Work out the finished part from the listing and answer in its coordinate system (mm). Face numbers are marked on the shaded views. A direction names the side the tool comes from. Give positions to 0.01 mm unless a question says otherwise; leave off trailing zeros. Order: outer loops, then holes, each group sorted by start corner. A loop starts at its lowest first (then second) coordinate and runs counter-clockwise, first axis right, second up. Notation, with made-up numbers: (-27, 5) - (-9, 5) arc R19 cw to (-9, 12) - close; hole circle Ø1 at (17.5, 63). An arc over 180 degrees is marked (long way). Put each result on its own line as item: value.
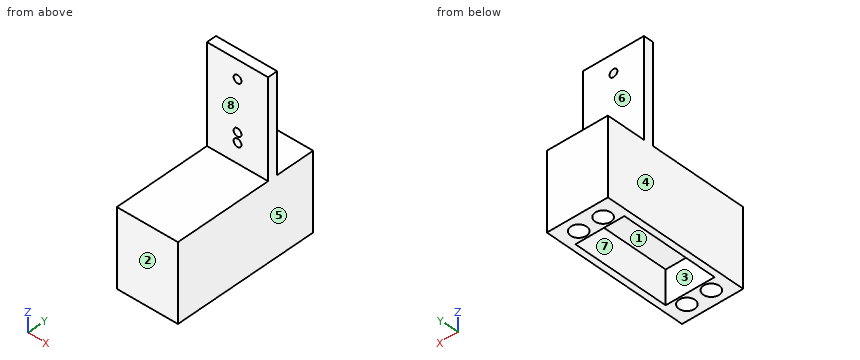
```python
from build123d import *

# Parameters (mm, degrees)
SKETCH1_W           = 27.5
SKETCH1_H           = 40
BOSS_EXTRUDE1_DEPTH = 12.5
SKETCH2_W           = 5.015
SKETCH2_H           = 40.03
SKETCH2_W_2         = 10
CUT_EXTRUDE1_DEPTH  = 13.765
SKETCH6_R           = 3.25
CUT_EXTRUDE2_DEPTH  = 12
SKETCH7_R           = 1.6
CUT_EXTRUDE3_DEPTH  = 61.763887302


with BuildPart() as part:
    # Sketch1 → Boss-Extrude1 (new, symmetric)
    with BuildSketch(Plane(origin=(0, 0, 0), x_dir=(0, 0, -1), z_dir=(1, 0, 0))):
        with Locations((17.75, 20)):
            Rectangle(SKETCH1_W, SKETCH1_H)
        Polygon((0, -10), (0, 30), (-40, 30), (-40, 34), (0, 34), (0, 50), (31.5, 50), (31.5, 40), (4, 40), (4, 0), (31.5, 0), (31.5, -10), align=None)
    extrude(amount=BOSS_EXTRUDE1_DEPTH, both=True)

    # Sketch2 → Cut-Extrude1 (cut, symmetric)
    with BuildSketch(Plane(origin=(0, 0, -31.5), x_dir=(-1, 0, 0), z_dir=(0, 0, -1))):
        with Locations((7.5075, 20)):
            Rectangle(SKETCH2_W, SKETCH2_H)
        with Locations((0, 20)):
            Rectangle(SKETCH2_W_2, SKETCH2_H)
        with Locations((-7.5075, 20)):
            Rectangle(SKETCH2_W, SKETCH2_H)
    extrude(amount=CUT_EXTRUDE1_DEPTH, both=True, mode=Mode.SUBTRACT)

    # Sketch6 → Cut-Extrude2 (cut)
    with BuildSketch(Plane(origin=(0, 0, -31.5), x_dir=(-1, 0, 0), z_dir=(0, 0, -1))):
        with Locations(Location((-5, 44, 0), (0, 0, 90))):
            Circle(SKETCH6_R)
        with Locations(Location((5, 44, 0), (0, 0, 90))):
            Circle(SKETCH6_R)
        with Locations(Location((5, -4, 0), (0, 0, 90))):
            Circle(SKETCH6_R)
        with Locations(Location((-5, -4, 0), (0, 0, 90))):
            Circle(SKETCH6_R)
    extrude(amount=-CUT_EXTRUDE2_DEPTH, mode=Mode.SUBTRACT)

    # Sketch7 → Cut-Extrude3 (cut, through all)
    with BuildSketch(Plane(origin=(0, 34, 0), x_dir=(1, 0, 0), z_dir=(0, 1, 0))):
        with Locations(Location((0, -32.5, 0), (0, 0, 270))):
            Circle(SKETCH7_R)
        with Locations(Location((0, -12, 0), (0, 0, 270))):
            Circle(SKETCH7_R)
        with Locations(Location((0, -8, 0), (0, 0, 270))):
            Circle(SKETCH7_R)
    extrude(amount=-CUT_EXTRUDE3_DEPTH, mode=Mode.SUBTRACT)


solid = part.part
```
(1) A tool of negligible diameter and unlimited length cuts with its end or side. For the marked faces 5, 6, 7 and 8, from which of +Z, -Z, +X, -X, +Y, -Y can it reach the whole face along a straight path? Write none if from no direction.
Geometry check:
face 5: +Z, -Z, +X, +Y, -Y
face 6: +Z, +X, -X, +Y
face 7: -Z
face 8: +Z, +X, -X, -Y
(2) Section D-D, the plane x = -5 is taken. Write down the section's boundary in (y, z) (3 decimals).
Geometry check:
outline: (-10, -31.5) - (-7.25, -31.5) - (-7.25, -19.5) - (-0.75, -19.5) - (-0.75, -31.5) - (-0.015, -31.5) - (-0.015, -17.735) - (40.015, -17.735) - (40.015, -31.5) - (40.75, -31.5) - (40.75, -19.5) - (47.25, -19.5) - (47.25, -31.5) - (50, -31.5) - (50, 0) - (34, 0) - (34, 40) - (30, 40) - (30, 0) - (-10, 0) - close
(3) Determine the mould class of the marked faces 1, 2, 3 and 4 for opening direction X: pulls with the +X half, pulls with the -X half, needs draft (parallel to the pull), parting line crosses it, or undercut.
Geometry check:
face 1: undercut
face 2: needs draft
face 3: undercut
face 4: pulls with the -X half
(4) Straight lines are drawn through the part: line 1 (Y direction, x = 0.5, z = -22.5) (3 decimals); line 2 (Z direction, x = 6.25, y = 14) (3 decimals); line 3 (Z direction, x = 1, y = -0.5). For each, find the intervals that lie inside material, in ascending order.
Geometry check:
line 1: y = -10 to -0.015, 40.015 to 50
line 2: z = -17.735 to 0
line 3: z = -31.5 to 0
(5) Given pin 1 (2 mm diameter, centred on x = -6, y = 43.5, fed in from -Z); pin 2 (12.5 mm diameter, centred on x = 4, z = 17.5, fed in from +Y); pin 3 (1 mm diameter, centred on x = 0.5, y = 23, fed in from -Z) (3 decimals), each flat-ended and moving along its own axis, determine where each tip first touches the part or whether it passes through.
Geometry check:
pin 1: stops at z = -19.5
pin 2: stops at y = 34
pin 3: stops at z = -17.735
(6) Section C-C, the plane y = 13 is taken. Write down the section's boundary in (x, z) (3 decimals), then the cut area to 3 significant figures.
Geometry check:
outline: (-12.5, -31.5) - (-10.015, -31.5) - (-10.015, -17.735) - (10.015, -17.735) - (10.015, -31.5) - (12.5, -31.5) - (12.5, 0) - (-12.5, 0) - close
area: 512 mm²
(7) Section B-B, the plane z = 12 is taken. Write down the section's boundary in (x, y).
Geometry check:
outline: (-12.5, 30) - (-1.6, 30) - (-1.6, 34) - (-12.5, 34) - close; (1.6, 30) - (12.5, 30) - (12.5, 34) - (1.6, 34) - close
(8) Section A-A, the plane x = 0 is taken. Write down the section's boundary in (y, z) (3 decimals), then the cut area to 3 significant figures.
Geometry check:
outline: (-10, -31.5) - (-0.015, -31.5) - (-0.015, -17.735) - (40.015, -17.735) - (40.015, -31.5) - (50, -31.5) - (50, 0) - (34, 0) - (34, 6.4) - (30, 6.4) - (30, 0) - (-10, 0) - close; (30, 9.6) - (34, 9.6) - (34, 10.4) - (30, 10.4) - close; (30, 13.6) - (34, 13.6) - (34, 30.9) - (30, 30.9) - close; (30, 34.1) - (34, 34.1) - (34, 40) - (30, 40) - close
area: 1,460 mm²
